```python
from build123d import *

# Parameters (mm, degrees)
SKETCH1_W               = 56.4
SKETCH1_H               = 56.4
BOSS_EXTRUDE1_DEPTH     = 4.2
SKETCH2_R               = 19.15
CUT_EXTRUDE1_DEPTH      = 1.6
SKETCH4_W               = 76.4
SKETCH4_H               = 76.4
BOSS_EXTRUDE2_DEPTH     = 5
SKETCH3_R               = 10
SKETCH3_R_2             = 2.5
CUT_EXTRUDE2_DEPTH      = 2.6
CUT_EXTRUDE2_DEPTH_BACK = 8.6
FILLET1_R               = 7
FILLET2_R               = 3
SKETCH5_R               = 2.5
CUT_EXTRUDE4_DEPTH      = 10
SKETCH6_R               = 20
CUT_EXTRUDE5_DEPTH      = 10


with BuildPart() as part:
    # Sketch1 → Boss-Extrude1 (new body)
    with BuildSketch(Plane.XY):
        Rectangle(SKETCH1_W, SKETCH1_H)
    extrude(amount=BOSS_EXTRUDE1_DEPTH)

    # Sketch2 → Cut-Extrude1 (cut)
    with BuildSketch(Plane.XY.offset(4.2)):
        Circle(SKETCH2_R)
    extrude(amount=-CUT_EXTRUDE1_DEPTH, mode=Mode.SUBTRACT)

    # Sketch4 → Boss-Extrude2 (add)
    with BuildSketch(Plane(origin=(0, 0, 0), x_dir=(-1, 0, 0), z_dir=(0, 0, -1))):
        Rectangle(SKETCH4_W, SKETCH4_H)
    extrude(amount=BOSS_EXTRUDE2_DEPTH)

    # Sketch3 → Cut-Extrude2 (cut, two sides)
    with BuildSketch(Plane.XY.offset(2.6)) as cut_extrude2_sk:
        Circle(SKETCH3_R)
        with Locations((23.55, -23.55)):
            Circle(SKETCH3_R_2)
        with Locations((-23.55, -23.55)):
            Circle(SKETCH3_R_2)
        with Locations((-23.55, 23.55)):
            Circle(SKETCH3_R_2)
        with Locations((23.55, 23.55)):
            Circle(SKETCH3_R_2)
    extrude(amount=CUT_EXTRUDE2_DEPTH, mode=Mode.SUBTRACT)
    extrude(cut_extrude2_sk.sketch, amount=-CUT_EXTRUDE2_DEPTH_BACK, mode=Mode.SUBTRACT)

    # Fillet1
    fillet1_edges = [part.edges().sort_by_distance(p)[0] for p in [
        (38.2, 38.2, -2.5),
        (38.2, -38.2, -2.5),
        (-38.2, -38.2, -2.5),
        (-38.2, 38.2, -2.5),
    ]]
    fillet(fillet1_edges, radius=FILLET1_R)

    # Fillet2
    fillet2_edges = [part.edges().sort_by_distance(p)[0] for p in [
        (28.2, -28.2, 2.1),
        (-28.2, -28.2, 2.1),
        (-28.2, 28.2, 2.1),
        (28.2, 28.2, 2.1),
    ]]
    fillet(fillet2_edges, radius=FILLET2_R)

    # Sketch5 → Cut-Extrude4 (cut)
    with BuildSketch(Plane(origin=(0, 0, -5), x_dir=(-1, 0, 0), z_dir=(0, 0, -1))):
        with Locations((-31.2, -31.2)):
            Circle(SKETCH5_R)
        with Locations((-31.2, 31.2)):
            Circle(SKETCH5_R)
        with Locations((31.2, 31.2)):
            Circle(SKETCH5_R)
        with Locations((31.2, -31.2)):
            Circle(SKETCH5_R)
    extrude(amount=-CUT_EXTRUDE4_DEPTH, mode=Mode.SUBTRACT)

    # Sketch6 → Cut-Extrude5 (cut)
    with BuildSketch(Plane(origin=(0, 0, -5), x_dir=(-1, 0, 0), z_dir=(0, 0, -1))):
        Circle(SKETCH6_R)
    extrude(amount=-CUT_EXTRUDE5_DEPTH, mode=Mode.SUBTRACT)


solid = part.part
```
Work out the finished part from the listing and answer in its coordinate system (mm). A direction names the side the tool comes from. Coordinates: 2 decimals unless noted, no trailing zeros. Loops run counter-clockwise (first coordinate to the right, second up) from the corner with the lowest first, then second, coordinate; pieces in that order, holes last.
1) Flat-ended cylindrical pins translate along their axes: pin 1 (1.5 mm diameter, centred on x = 16.5, y = -7.5, fed in from -Z); pin 2 (3.5 mm diameter, centred on x = -0.5, z = 2.5, fed in from -Y); pin 3 (2 mm diameter, centred on y = 11.5, z = 2.5, fed in from +X); pin 4 (8 mm diameter, centred on x = 31.2, y = 31.2, fed in from +Z). Find the tip coordinate at first contact, or state that the pin passes through.
Results:
pin 1: passes through
pin 2: stops at y = -28.2
pin 3: stops at x = 28.2
pin 4: stops at z = 0
2) For faces 4 (the flat face through (28.2, 0, 2)), 5 (the cylindrical face through (27.3, 27.34, 2.13)), 6 (the flat face through (-33, 1, 0)), determine the directions among +Z, -Z, +X, -X, +Y, -Y from which every point of the face is accessible in a straight line to the end or side of a thin tool.
Results:
face 4: +Z, +X, +Y, -Y
face 5: +Z, +X, +Y
face 6: +Z
3) Section C-C (z = -3.5) is taken. Give the number of separate pieces and of enclosed holes in the cut face, plus the area to 3 significant figures.
Results:
separate pieces: 1
enclosed holes: 9
area: 4,380 mm2
4) Section B-B (y = 0) is taken. Give the vertices of the cut face in (x, z).
Results:
outline: (-38.2, -5) - (-20, -5) - (-20, 4.2) - (-28.2, 4.2) - (-28.2, 0) - (-38.2, 0) - close; (20, -5) - (38.2, -5) - (38.2, 0) - (28.2, 0) - (28.2, 4.2) - (20, 4.2) - close
5) Section A-A (x = 23.55) is taken. Give the vertices of the cut face in (y, z), plus the area to 3 significant figures.
Results:
outline: (-38.2, -5) - (-26.05, -5) - (-26.05, 4.2) - (-28.2, 4.2) - (-28.2, 0) - (-38.2, 0) - close; (-21.05, -5) - (21.05, -5) - (21.05, 4.2) - (-21.05, 4.2) - close; (26.05, -5) - (38.2, -5) - (38.2, 0) - (28.2, 0) - (28.2, 4.2) - (26.05, 4.2) - close
area: 527 mm2
6) For a pull along X with two mould halves and no side action, classify faces 1 (the cylindrical face through (27.34, -27.3, 2.13)), 2 (the flat face through (0, -28.2, 2)), 3 (the cylindrical face through (-24.09, -25.99, -0.34)) as +X half, -X half, draft (parallel to the pull), parting line (faces both ways), or undercut.
Results:
face 1: +X half
face 2: draft
face 3: undercut
7) Consider probe 1 along Y at (x, z) = (-31.2, -1.75); probe 2 along X at (y, z) = (23.55, 0.25); probe 3 along Y at (x, z) = (-23.5, -1.5). Determine where each line is inside the solid, lowest interval first.
Results:
probe 1: y = -38.2 to -33.7, -28.7 to 28.7, 33.7 to 38.2
probe 2: x = -28.2 to -26.05, -21.05 to 21.05, 26.05 to 28.2
probe 3: y = -38.2 to -26.05, -21.05 to 21.05, 26.05 to 38.2
